Source: CAD feature listing. Evaluate the final solid. Frame: model axes, mm. Face numbers are marked on the shaded views. A direction names the side the tool comes from. Give positions to 0.01 mm unless a question says otherwise; leave off trailing zeros. Loops run counter-clockwise (first coordinate to the right, second up) from the corner with the lowest first, then second, coordinate; pieces in that order, holes last. Notation, with made-up numbers: (52, 6.25) -> (62, 6.25) arc R20 cw to (62, 11.25) -> close; hole circle Ø1 at (49, 85). An arc over 180 degrees is marked (long way). Put each result on its own line as item: value.
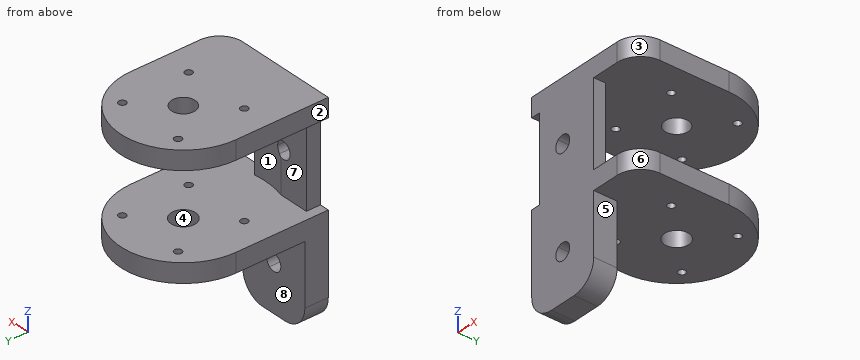
```python
from build123d import *

# Parameters (mm, degrees)
SKETCH1_R                      = 16.934647101
SKETCH1_R_2                    = 1
SKETCH1_R_3                    = 7.5
BOSS_EXTRUDE1_DEPTH            = 5.08
BOSS_EXTRUDE2_START            = -5.08
BOSS_EXTRUDE2_DEPTH            = 5.08
SKETCH3_W                      = 20
SKETCH3_H                      = 6.35
BOSS_EXTRUDE3_DEPTH            = 50.8
BOSS_EXTRUDE4_START            = -25.4
BOSS_EXTRUDE4_DEPTH            = 2.597534174
SKETCH5_R                      = 3.302
CUT_EXTRUDE1_DEPTH             = 50.8
SKETCH6_W                      = 13.869294202
SKETCH6_H                      = 2.597534174
BOSS_EXTRUDE5_DEPTH            = 6.35
CUT_EXTRUDE2_DEPTH             = 50.8
BOSS_EXTRUDE7_START            = 2.54
SKETCH8_R                      = 3.302
BOSS_EXTRUDE7_DEPTH            = 2.54
CUT_EXTRUDE3_REACH             = 55.758
SKETCH10_R                     = 22.133090672
CUT_EXTRUDE3_DIRECTION_2_REACH = 55.758
FILLET1_R                      = 6.35
FILLET3_R                      = 6.35
SKETCH11_R                     = 1
CUT_EXTRUDE4_DEPTH             = 45.770838885
BOSS_EXTRUDE8_START            = -5.08
SKETCH12_R                     = 7.5
SKETCH12_R_2                   = 3.175
BOSS_EXTRUDE8_DEPTH            = 5.08
SKETCH13_W                     = 14.910856388
SKETCH13_H                     = 22.802465826
SKETCH13_W_2                   = 5.089143612
CUT_EXTRUDE5_DEPTH             = 2.54
SKETCH14_W                     = 22.802465826
SKETCH14_H                     = 1.813273425
SKETCH14_H_2                   = 0.683329188
SKETCH14_H_3                   = 3.126670812
CUT_EXTRUDE6_DEPTH             = 2.54


# Read off the part's stored shape, not the designer's step: Boss-Extrude4
with BuildPart() as part:
    # Sketch1 → Boss-Extrude1 (new body)
    with BuildSketch(Plane.XY):
        Circle(SKETCH1_R)
        with Locations((8.980256121, 8.980256121)):
            Circle(SKETCH1_R_2, mode=Mode.SUBTRACT)
        with Locations((8.980256121, -8.980256121)):
            Circle(SKETCH1_R_2, mode=Mode.SUBTRACT)
        with Locations((-8.980256121, -8.980256121)):
            Circle(SKETCH1_R_2, mode=Mode.SUBTRACT)
        with Locations((-8.980256121, 8.980256121)):
            Circle(SKETCH1_R_2, mode=Mode.SUBTRACT)
        Circle(SKETCH1_R_3, mode=Mode.SUBTRACT)
    extrude(amount=BOSS_EXTRUDE1_DEPTH)

    # Sketch2 → Boss-Extrude2 (add)
    with BuildSketch(Plane.XY.offset(5.08).offset(BOSS_EXTRUDE2_START)):
        with BuildLine():
            ThreePointArc((16.934647101, 0), (0, -16.934647101), (-16.934647101, 0))
            Line((-16.934647101, 0), (-16.934647101, -25.046463564))
            Line((-16.934647101, -25.046463564), (16.934647101, -25.046463564))
            Line((16.934647101, -25.046463564), (16.934647101, 0))
        make_face()
    extrude(amount=BOSS_EXTRUDE2_DEPTH)

    # Sketch3 → Boss-Extrude3 (add)
    with BuildSketch(Plane(origin=(0, 0, 0), x_dir=(-1, 0, 0), z_dir=(0, 0, -1))):
        with Locations((6.934647101, -21.871463564)):
            Rectangle(SKETCH3_W, SKETCH3_H)
    extrude(amount=BOSS_EXTRUDE3_DEPTH)

    # Boss-Extrude4 outline → Boss-Extrude4 (add)
    with BuildSketch(Plane.XY.offset(BOSS_EXTRUDE4_START)):
        with BuildLine():
            ThreePointArc((16.934647101, 0), (0, 16.934647101), (-16.934647101, 0))
            Line((-16.934647101, 0), (-16.934647101, -18.696463564))
            Line((-16.934647101, -18.696463564), (16.934647101, -18.696463564))
            Line((16.934647101, -18.696463564), (16.934647101, 0))
        make_face()
    extrude(amount=BOSS_EXTRUDE4_DEPTH)

    # Sketch5 → Cut-Extrude1 (cut)
    with BuildSketch(Plane(origin=(0, 0, -25.4), x_dir=(-1, 0, 0), z_dir=(0, 0, -1))):
        Circle(SKETCH5_R)
    extrude(amount=-CUT_EXTRUDE1_DEPTH, mode=Mode.SUBTRACT)

    # Sketch6 → Boss-Extrude5 (add)
    with BuildSketch(Plane.XZ.offset(18.696463564)):
        with Locations((10, -24.101232913)):
            Rectangle(SKETCH6_W, SKETCH6_H)
    extrude(amount=BOSS_EXTRUDE5_DEPTH)

    # Sketch7 → Cut-Extrude2 (cut)
    with BuildSketch(Plane(origin=(0, -18.696463564, 0), x_dir=(1, 0, 0), z_dir=(0, 1, 0))):
        with BuildLine():
            ThreePointArc((-4.684647101, 11.401232913), (-4.885171568, 12.329753263), (-5.451002692, 13.092770459))
            Line((-5.451002692, 13.092770459), (-8.418291509, 9.709695367))
            ThreePointArc((-8.418291509, 9.709695367), (-6.00612675, 9.35175738), (-4.684647101, 11.401232913))
        make_face()
        with BuildLine():
            Line((-8.418291509, 9.709695367), (-5.451002692, 13.092770459))
            ThreePointArc((-5.451002692, 13.092770459), (-8.626184647, 12.884877321), (-8.418291509, 9.709695367))
        make_face()
        with BuildLine():
            ThreePointArc((-5.542705151, 39.867766276), (-8.702413377, 39.49194195), (-8.32658905, 36.332233724))
            Line((-8.32658905, 36.332233724), (-5.542705151, 39.867766276))
        make_face()
        with BuildLine():
            Line((-5.542705151, 39.867766276), (-8.32658905, 36.332233724))
            ThreePointArc((-8.32658905, 36.332233724), (-5.952142492, 36.075849637), (-4.684647101, 38.1))
            ThreePointArc((-4.684647101, 38.1), (-4.910496737, 39.082504609), (-5.542705151, 39.867766276))
        make_face()
    extrude(amount=-CUT_EXTRUDE2_DEPTH, mode=Mode.SUBTRACT)

    # Sketch8 → Boss-Extrude7 (add)
    with BuildSketch(Plane(origin=(0, 0, -25.4), x_dir=(-1, 0, 0), z_dir=(0, 0, -1)).offset(BOSS_EXTRUDE7_START)):
        with BuildLine():
            Line((-16.934647101, 0), (-16.934647101, -25.046463564))
            Line((-16.934647101, -25.046463564), (-3.065352899, -25.046463564))
            Line((-3.065352899, -25.046463564), (-3.065352899, -18.696463564))
            Line((-3.065352899, -18.696463564), (16.934647101, -18.696463564))
            Line((16.934647101, -18.696463564), (16.934647101, 0))
            ThreePointArc((16.934647101, 0), (0, 16.934647101), (-16.934647101, 0))
        make_face()
        Circle(SKETCH8_R, mode=Mode.SUBTRACT)
    extrude(amount=-BOSS_EXTRUDE7_DEPTH)

    # Cut-Extrude3: up to this face of the body (flat: up to its plane)
    cut_extrude3_end = Plane(part.part.faces().sort_by_distance((0.774222072, -4.051019625, -22.802465826))[0])
    # Sketch10 → Cut-Extrude3 (cut, up to the picked face)
    with BuildSketch(Plane.XY.offset(-6.35), mode=Mode.PRIVATE) as cut_extrude3_sk1:
        Circle(SKETCH10_R)
    cut_extrude3_tool1 = split(extrude(cut_extrude3_sk1.sketch, amount=-CUT_EXTRUDE3_REACH, mode=Mode.PRIVATE), bisect_by=cut_extrude3_end, keep=Keep.BOTH, mode=Mode.PRIVATE)
    add(cut_extrude3_tool1.solids().sort_by(Axis((0, 0, -6.35), (0, 0, -1)))[0], mode=Mode.SUBTRACT)

    # Cut-Extrude3 direction 2: up to this face of the body (flat: up to its plane)
    cut_extrude3_direction_2_end = Plane(part.part.faces().sort_by_distance((16.395245326, -12.523231782, 0))[0])
    # Sketch10 → Cut-Extrude3 direction 2 (cut, up to the picked face)
    with BuildSketch(Plane.XY.offset(-6.35), mode=Mode.PRIVATE) as cut_extrude3_direction_2_sk1:
        Circle(SKETCH10_R)
    cut_extrude3_direction_2_tool1 = split(extrude(cut_extrude3_direction_2_sk1.sketch, amount=CUT_EXTRUDE3_DIRECTION_2_REACH, mode=Mode.PRIVATE), bisect_by=cut_extrude3_direction_2_end, keep=Keep.BOTH, mode=Mode.PRIVATE)
    add(cut_extrude3_direction_2_tool1.solids().sort_by(Axis((0, 0, -6.35), (0, 0, 1)))[0], mode=Mode.SUBTRACT)

    # Fillet1
    fillet1_edges = [part.edges().sort_by_distance(p)[0] for p in [
        (16.934647101, -25.046463564, 2.54),
        (16.934647101, -25.046463564, -25.371232913),
    ]]
    fillet(fillet1_edges, radius=FILLET1_R)

    # Fillet3
    fillet3_edges = [part.edges().sort_by_distance(p)[0] for p in [
        (-16.934647101, -21.871463564, -50.8),
        (3.065352899, -21.871463564, -50.8),
    ]]
    fillet(fillet3_edges, radius=FILLET3_R)

    # Sketch11 → Cut-Extrude4 (cut, through all)
    with BuildSketch(Plane(origin=(0, 0, -27.94), x_dir=(-1, 0, 0), z_dir=(0, 0, -1))):
        with Locations(Location((-8.980256121, -8.980256121, 0), (0, 0, 180))):
            Circle(SKETCH11_R)
        with Locations(Location((-8.980256121, 8.980256121, 0), (0, 0, 180))):
            Circle(SKETCH11_R)
        with Locations(Location((8.980256121, -8.980256121, 0), (0, 0, 180))):
            Circle(SKETCH11_R)
        with Locations(Location((8.980256121, 8.980256121, 0), (0, 0, 180))):
            Circle(SKETCH11_R)
    extrude(amount=-CUT_EXTRUDE4_DEPTH, mode=Mode.SUBTRACT)

    # Sketch12 → Boss-Extrude8 (add)
    with BuildSketch(Plane.XY.offset(5.08).offset(BOSS_EXTRUDE8_START)):
        Circle(SKETCH12_R)
        Circle(SKETCH12_R_2, mode=Mode.SUBTRACT)
    extrude(amount=BOSS_EXTRUDE8_DEPTH)

    # Sketch13 → Cut-Extrude5 (cut)
    with BuildSketch(Plane(origin=(0, -18.696463564, 0), x_dir=(1, 0, 0), z_dir=(0, 1, 0))):
        with Locations((-4.390075295, 11.401232913)):
            Rectangle(SKETCH13_W, SKETCH13_H)
        with Locations((-14.390075295, 11.401232913)):
            Rectangle(SKETCH13_W_2, SKETCH13_H)
    extrude(amount=-CUT_EXTRUDE5_DEPTH, mode=Mode.SUBTRACT)

    # Sketch14 → Cut-Extrude6 (cut)
    with BuildSketch(Plane.ZY.offset(16.934647101)):
        with Locations((-11.401232913, -20.329826852)):
            Rectangle(SKETCH14_W, SKETCH14_H)
        with Locations((-11.401232913, -21.578128158)):
            Rectangle(SKETCH14_W, SKETCH14_H_2)
        with Locations((-11.401232913, -23.483128158)):
            Rectangle(SKETCH14_W, SKETCH14_H_3)
    extrude(amount=-CUT_EXTRUDE6_DEPTH, mode=Mode.SUBTRACT)


solid = part.part
```
(1) Draft query along X for the marked faces 1, 2 and 3. Return one class per face: released by +X, released by -X, zero draft, split by the parting line, or undercut.
Calculated:
face 1: undercut
face 2: released by -X
face 3: released by +X
(2) Reachability of the marked faces 4, 5, 6, 7 and 8 from +Z, -Z, +X, -X, +Y, -Y: full face, straight path, thin tool, end or side. Return the list, or none.
Calculated:
face 4: -Z
face 5: -Z, +X, +Y, -Y
face 6: +Z, -Z, +X, -Y
face 7: +X, -X, +Y
face 8: -Z, +X, -X, +Y
(3) First-contact query: P1, Ø1, axis at x = 11.5, y = -14, coming from the -Z side; P2, Ø2.5, axis at y = -23.5, z = -16.5, coming from the +X side; P3, Ø1.1, axis at y = -24, z = -10.5, coming from the -X side; P4, Ø1.6, axis at x = -8.98, y = 8.98, coming from the -Z side. Flat tips, straight axial feed; report the tip coordinate or a pass-through.
Calculated:
P1: stops at z = -27.94
P2: stops at x = 3.07
P3: stops at x = -14.39
P4: passes through
(4) Section B-B on x = 12. Return loops of the section in (y, z).
Calculated:
outline: (-24.89, -27.94) -> (11.95, -27.94) -> (11.95, -22.8) -> (-24.89, -22.8) -> close; (-24.89, 0) -> (11.95, 0) -> (11.95, 5.08) -> (-24.89, 5.08) -> close
(5) Section A-A on y = -5.5. Return loops of the section in (x, z).
Calculated:
outline: (-16.93, -27.94) -> (16.93, -27.94) -> (16.93, -22.8) -> (-16.93, -22.8) -> close; (-16.93, 0) -> (16.93, 0) -> (16.93, 5.08) -> (-16.93, 5.08) -> close
(6) Section C-C on x = 0. Return loops of the section in (y, z) (3 decimals), then the cut area to 3 significant figures.
Calculated:
outline: (-25.046, -49.884) -> (-18.696, -49.884) -> (-18.696, -27.94) -> (-3.302, -27.94) -> (-3.302, -22.802) -> (-22.133, -22.802) -> (-22.133, 0) -> (-3.175, 0) -> (-3.175, 5.08) -> (-25.046, 5.08) -> close; (3.175, 0) -> (16.935, 0) -> (16.935, 5.08) -> (3.175, 5.08) -> close; (3.302, -27.94) -> (16.935, -27.94) -> (16.935, -22.802) -> (3.302, -22.802) -> close
area: 569 mm²
(7) Line query: probe 1 along Z at (x, y) = (14.5, 7); probe 2 along Y at (x, z) = (0, 1.25) (3 decimals); probe 3 along Y at (x, z) = (-9.5, -6). Output: solid intervals per line, ascending. Write a range as from..to.
Calculated:
probe 1: z = -27.94..-22.8, 0..5.08
probe 2: y = -25.046..-3.175, 3.175..16.935
probe 3: y = -25.05..-21.24
(8) Section D-D on y = 1. Return loops of the section in (x, z), then the cut area to 3 significant figures.
Calculated:
outline: (-16.91, -27.94) -> (-3.15, -27.94) -> (-3.15, -22.8) -> (-16.91, -22.8) -> close; (-16.91, 0) -> (-3.01, 0) -> (-3.01, 5.08) -> (-16.91, 5.08) -> close; (3.01, 0) -> (16.91, 0) -> (16.91, 5.08) -> (3.01, 5.08) -> close; (3.15, -27.94) -> (16.91, -27.94) -> (16.91, -22.8) -> (3.15, -22.8) -> close
area: 283 mm²
